from build123d import *

# Parameters (mm, degrees)
BOSS_EXTRUDE1_DEPTH = 10
SKETCH2_R           = 2.1
CUT_EXTRUDE1_DEPTH  = 9
FILLET1_R           = 4


with BuildPart() as part:
    # Sketch1 → Boss-Extrude1 (new body)
    with BuildSketch(Plane(origin=(0, 0, 0), x_dir=(1, 0, 0), z_dir=(0, 1, 0))):
        with BuildLine():
            Line((-38, -8), (38, -8))
            Line((38, -8), (38, 0))
            Line((38, 0), (26, 0))
            ThreePointArc((26, 0), (22.5, -3.5), (19, 0))
            Line((19, 0), (-19, 0))
            ThreePointArc((-19, 0), (-22.5, -3.5), (-26, 0))
            Line((-26, 0), (-38, 0))
            Line((-38, 0), (-38, -8))
        make_face()
    extrude(amount=BOSS_EXTRUDE1_DEPTH)

    # Sketch2 → Cut-Extrude1 (cut, through all)
    with BuildSketch(Plane(origin=(0, 0, 0), x_dir=(-1, 0, 0), z_dir=(0, 0, -1))):
        with Locations((32, 5)):
            Circle(SKETCH2_R)
        with Locations((-32, 5)):
            Circle(SKETCH2_R)
        with Locations((0, 5)):
            Circle(SKETCH2_R)
    extrude(amount=-CUT_EXTRUDE1_DEPTH, mode=Mode.SUBTRACT)

    # Fillet1
    fillet1_edges = [part.edges().sort_by_distance(p)[0] for p in [
        (38, 0, 4),
        (-38, 0, 4),
        (38, 10, 4),
        (-38, 10, 4),
    ]]
    fillet(fillet1_edges, radius=FILLET1_R)


solid = part.part
Geometry: final body of the model. Coordinates: model frame, mm. Round coordinates to 2 decimals unless told otherwise and drop trailing zeros. Loops run counter-clockwise (first coordinate to the right, second up) from the corner with the lowest first, then second, coordinate; pieces in that order, holes last. Notation, with made-up numbers: M 35,6.25 L 41,6.25 A25 cw 41,27.25 Z; hole C 41,-4.75 d10. An arc over 180 degrees is marked long. One line per question, with ' | ' between items.
(1) Pull-direction query (X, two-part tool) for faces 1 (the cylindrical face through (36.797, 1.141, 3.944)), 2 (the cylindrical face through (22.6, 4.9, 3.5)), 3 (the flat face through (-30.6, 7.2, 0)), 4 (the cylindrical face through (-29.9, 5.09, 3.94)); classes: +X half, -X half, draft (parallel to the pull), parting line (faces both ways), or undercut.
Check result:
face 1: +X half | face 2: undercut | face 3: draft | face 4: undercut
(2) Cut plane C-C on z = 4.5. Return the cut outline in (x, y).
Check result:
outline: M -38,4 A4 ccw -34,0 L 34,0 A4 ccw 38,4 L 38,6 A4 ccw 34,10 L -34,10 A4 ccw -38,6 Z; hole C -32,5 d4.2; hole C 0,5 d4.2; hole C 32,5 d4.2
(3) Cut plane A-A on z = 1. Return the cut outline in (x, y).
Check result:
outline: M -38,4 A4 ccw -34,0 L -25.85,0 L -25.85,10 L -34,10 A4 ccw -38,6 Z; M -19.15,0 L 19.15,0 L 19.15,10 L -19.15,10 Z; M 25.85,0 L 34,0 A4 ccw 38,4 L 38,6 A4 ccw 34,10 L 25.85,10 Z; hole C -32,5 d4.2; hole C 0,5 d4.2; hole C 32,5 d4.2
(4) Cut plane B-B on x = -32. Return the cut outline in (y, z).
Check result:
outline: M 0,0 L 2.9,0 L 2.9,8 L 0,8 Z; M 7.1,0 L 10,0 L 10,8 L 7.1,8 Z
(5) Material intervals for line 1 along X through (y, z) = (5.25, 5.5); line 2 along X through (y, z) = (3.75, 4.75); line 3 along Y through (x, z) = (32, 2), sorted ascending. Write a range as from..to.
Check result:
line 1: x = -38..-34.09, -29.91..-2.09, 2.09..29.91, 34.09..38 | line 2: x = -37.99..-33.69, -30.31..-1.69, 1.69..30.31, 33.69..37.99 | line 3: y = 0..2.9, 7.1..10
(6) Cut plane D-D on y = 8.5. Return the cut outline in (x, z), plus the area to 3 significant figures.
Check result:
outline: M -37.12,0 L -26,0 A3.5 cw -19,0 L 19,0 A3.5 cw 26,0 L 37.12,0 L 37.12,8 L -37.12,8 Z | area: 555 mm2
